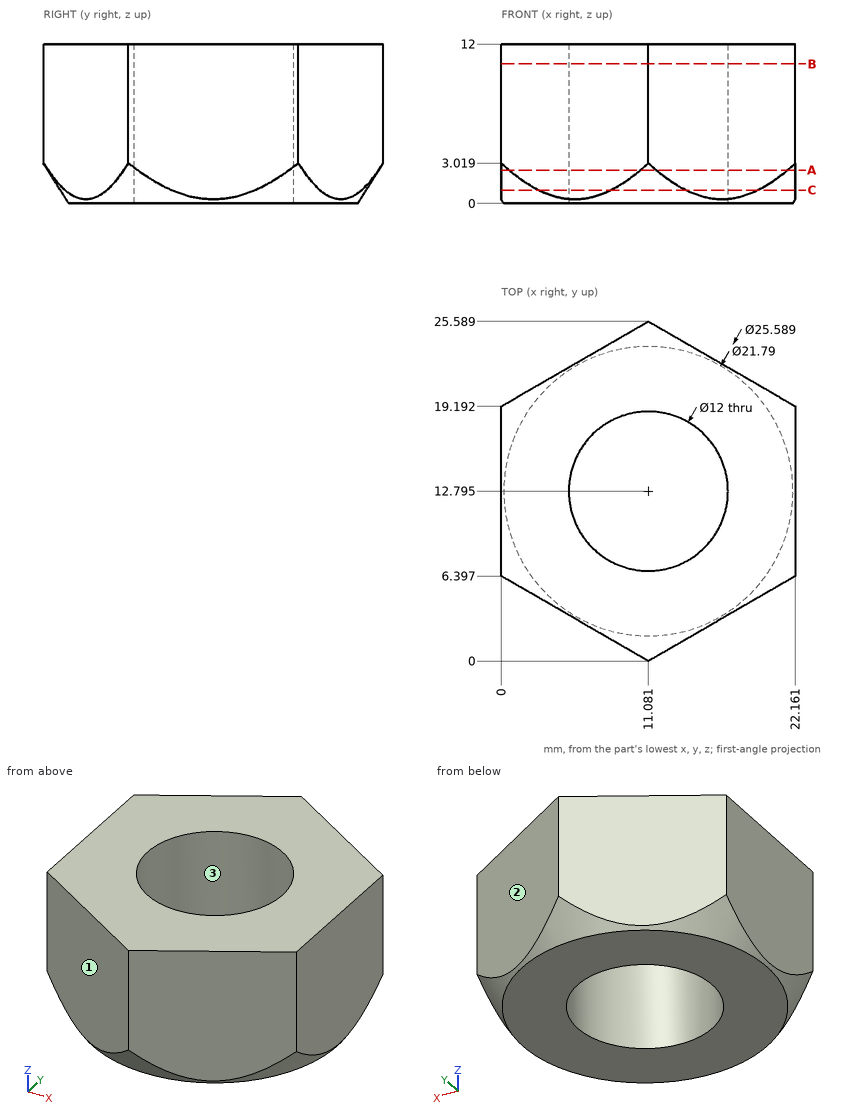
Geometry check sheet. Reference: drawing and pictorial views, mm from the part's lowest x, y, z. Give positions to 0.01 mm unless a question says otherwise; leave off trailing zeros. Order: outer loops, then holes, each group sorted by start corner. A loop starts at its lowest first (then second) coordinate and runs counter-clockwise, first axis right, second up. Notation, with made-up numbers: (-14, 32) - (44, 32) arc R28 cw to (44, 65) - close; hole circle Ø3 at (-7.5, -26). An arc over 180 degrees is marked (long way). Use one line per item in the form item = value.
1) Sectioned sample at C-C (z = 1). Record the boundary of the cut face in (x, y) (1 decimal), and give its area (3 significant figures).
Working result:
outline = (0, 9.6) arc R11.5 ccw to (2.8, 4.8) - (8.3, 1.6) arc R11.5 ccw to (13.9, 1.6) - (19.4, 4.8) arc R11.5 ccw to (22.2, 9.6) - (22.2, 16) arc R11.5 ccw to (19.4, 20.8) - (13.9, 24) arc R11.5 ccw to (8.3, 24) - (2.8, 20.8) arc R11.5 ccw to (0, 16) - close; hole circle Ø12 at (11.1, 12.8)
area = 293 mm^2
2) Sectioned sample at A-A (z = 2.5). Record the boundary of the cut face in (x, y) (1 decimal).
Working result:
outline = (0, 7.1) arc R12.5 ccw to (0.6, 6.1) - (10.5, 0.3) arc R12.5 ccw to (11.7, 0.3) - (21.6, 6.1) arc R12.5 ccw to (22.2, 7.1) - (22.2, 18.5) arc R12.5 ccw to (21.6, 19.5) - (11.7, 25.2) arc R12.5 ccw to (10.5, 25.2) - (0.6, 19.5) arc R12.5 ccw to (0, 18.5) - close; hole circle Ø12 at (11.1, 12.8)
3) Depth check by flat-ended pin: pin 1 Ø1 at (x, z) = (19, 6) entering from -Y (1 decimal). Enter the tip coordinate at first touch or a pass-through.
Working result:
pin_1 = 4.3
4) Sectioned sample at B-B (z = 10.5). Record the boundary of the cut face in (x, y) (1 decimal).
Working result:
outline = (0, 6.4) - (11.1, 0) - (22.2, 6.4) - (22.2, 19.2) - (11.1, 25.6) - (0, 19.2) - close; hole circle Ø12 at (11.1, 12.8)
5) Draft check along X on the marked faces 1, 2 and 3. Enter one of: released by +X, released by -X, zero draft, split by the parting line, or undercut.
Working result:
face_1 = released by -X
face_2 = released by +X
face_3 = undercut
6) Material ranges on probe 1 along X at (y, z) = (13, 8.75) (1 decimal); probe 2 along Y at (x, z) = (6.5, 2.25) (1 decimal); probe 3 along Y at (x, z) = (10.75, 10.5) (1 decimal), recorded low to high. Write a range as from..to.
Working result:
probe_1 = 0..5.1, 17.1..22.2
probe_2 = 2.6..8.9, 16.7..22.9
probe_3 = 0.2..6.8, 18.8..25.4
